Source: CAD feature listing. Evaluate the final solid. Frame: model axes, mm. Face numbers are marked on the shaded views. A direction names the side the tool comes from. Give positions to 0.01 mm unless a question says otherwise; leave off trailing zeros. Loops run counter-clockwise (first coordinate to the right, second up) from the corner with the lowest first, then second, coordinate; pieces in that order, holes last.
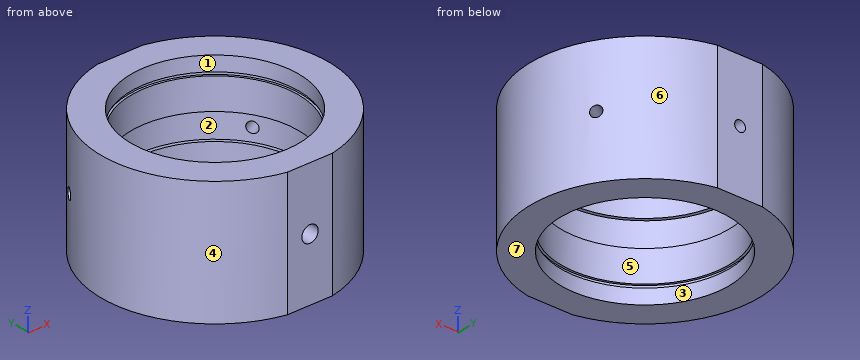
from build123d import *

# Parameters (mm, degrees)
SKETCH_2_W                       = 64.02174429
SKETCH_2_H                       = 9.248919907
CUT_EXTRUDE_1_DEPTH              = 49
HOLE_WIZARD_M4_2_D               = 3.3
HOLE_WIZARD_M4_2_DEPTH           = 5.5
HOLE_WIZARD_M4_2_TIP             = 0.991420021
HOLE_WIZARD_M6_2_D               = 5
HOLE_WIZARD_M6_2_DEPTH           = 5.5
HOLE_WIZARD_M6_2_TIP             = 1.502151548
HOLE_WIZARD_M4_3_D               = 3.3
HOLE_WIZARD_M4_3_DEPTH           = 10.1
HOLE_WIZARD_M4_3_TIP             = 0.991420021
HOLE_WIZARD_M4_3_ON_FACE_2_D     = 3.3
HOLE_WIZARD_M4_3_ON_FACE_2_DEPTH = 10.1
HOLE_WIZARD_M4_3_ON_FACE_2_TIP   = 0.991420021


with BuildPart() as part:
    # 草图1 → 旋转1 (revolve)
    with BuildSketch(Plane(origin=(0, 0, 0), x_dir=(1, 0, 0), z_dir=(0, 1, 0)), mode=Mode.PRIVATE) as revolve_1_sk:
        Polygon((34.5, 19), (34.5, -19), (25.5, -19), (25.5, -14.5), (26.1, -14.5), (26.1, -13.5), (25.4, -13.5), (25.4, -4), (26.5, -4), (26.5, 4), (25.4, 4), (25.4, 13.5), (26.1, 13.5), (26.1, 14.5), (25.5, 14.5), (25.5, 19), align=None)
    revolve(revolve_1_sk.sketch.rotate(Axis((0, 0, -31.9390681), (0, 0, 1)), 180), axis=Axis((0, 0, -31.9390681), (0, 0, 1)))  # turned: the seam where the file's is

    # 草图2 → 切除-拉伸1 (cut)
    with BuildSketch(Plane.XY.offset(19)):
        with Locations((-1.141100508, 38.424459954)):
            Rectangle(SKETCH_2_W, SKETCH_2_H)
        with Locations((-1.141100508, -38.424459954)):
            Rectangle(SKETCH_2_W, SKETCH_2_H)
    extrude(amount=-CUT_EXTRUDE_1_DEPTH, mode=Mode.SUBTRACT)

    # M4 螺纹孔2
    with Locations(Plane(origin=(0, 33.8, 0), x_dir=(1, 0, 0), z_dir=(0, 1, 0))):
        with Locations((0, 0)):
            Hole(HOLE_WIZARD_M4_2_D / 2, depth=HOLE_WIZARD_M4_2_DEPTH)
            with Locations((0, 0, -(HOLE_WIZARD_M4_2_DEPTH + HOLE_WIZARD_M4_2_TIP / 2))):  # 118° drill point
                Cone(0, HOLE_WIZARD_M4_2_D / 2, HOLE_WIZARD_M4_2_TIP, mode=Mode.SUBTRACT)

    # M6 螺纹孔2
    with Locations(Plane(origin=(0, -33.8, 0), x_dir=(-1, 0, 0), z_dir=(0, -1, 0))):
        with Locations((0, 0)):
            Hole(HOLE_WIZARD_M6_2_D / 2, depth=HOLE_WIZARD_M6_2_DEPTH)
            with Locations((0, 0, -(HOLE_WIZARD_M6_2_DEPTH + HOLE_WIZARD_M6_2_TIP / 2))):  # 118° drill point
                Cone(0, HOLE_WIZARD_M6_2_D / 2, HOLE_WIZARD_M6_2_TIP, mode=Mode.SUBTRACT)

    # M4 螺纹孔3
    with Locations(Plane(origin=(29.877876431, 17.25, 0), x_dir=(-0.5, 0.866025404, 0), z_dir=(0.866025404, 0.5, 0))):
        with Locations((0, 0)):
            Hole(HOLE_WIZARD_M4_3_D / 2, depth=HOLE_WIZARD_M4_3_DEPTH)
            with Locations((0, 0, -(HOLE_WIZARD_M4_3_DEPTH + HOLE_WIZARD_M4_3_TIP / 2))):  # 118° drill point
                Cone(0, HOLE_WIZARD_M4_3_D / 2, HOLE_WIZARD_M4_3_TIP, mode=Mode.SUBTRACT)

    # M4 螺纹孔3 on face 2
    with Locations(Plane(origin=(-29.877876431, 17.25, 0), x_dir=(-0.500000175, -0.866025303, 0), z_dir=(-0.866025303, 0.500000175, 0))):
        with Locations((0, 0)):
            Hole(HOLE_WIZARD_M4_3_ON_FACE_2_D / 2, depth=HOLE_WIZARD_M4_3_ON_FACE_2_DEPTH)
            with Locations((0, 0, -(HOLE_WIZARD_M4_3_ON_FACE_2_DEPTH + HOLE_WIZARD_M4_3_ON_FACE_2_TIP / 2))):  # 118° drill point
                Cone(0, HOLE_WIZARD_M4_3_ON_FACE_2_D / 2, HOLE_WIZARD_M4_3_ON_FACE_2_TIP, mode=Mode.SUBTRACT)


solid = part.part
1) Reachability of the marked faces 1, 2 and 3 from +Z, -Z, +X, -X, +Y, -Y: full face, straight path, thin tool, end or side. Return the list, or none.
Checks:
face 1: +Z
face 2: none
face 3: -Z
2) Pull-direction query (X, two-part tool) for the marked faces 4, 5, 6 and 7; classes: released by +X, released by -X, zero draft, split by the parting line, or undercut.
Checks:
face 4: released by -X
face 5: undercut
face 6: released by +X
face 7: zero draft
3) Ray query, probe 1 along Z at (x, y) = (0, 32.5); probe 2 along Y at (x, z) = (0, 13); probe 3 along Z at (x, y) = (-26, -4). Return the intervals inside material, ascending.
Checks:
probe 1: z = -19 to -1.65, 1.65 to 19
probe 2: y = -33.8 to -25.4, 25.4 to 33.8
probe 3: z = -19 to -4, 4 to 19
4) Contact query for flat-ended pins moving along their axis: P1, Ø6, axis at y = -7.5, z = 10.5, coming from the +X side; P2, Ø12, axis at y = -19.5, z = 8.5, coming from the -X side; P3, Ø4, axis at y = -23.5, z = -0.5, coming from the +X side. Output: stop coordinate, or through.
Checks:
P1: stops at x = 34.21
P2: stops at x = -31.75
P3: stops at x = 26.98
5) Cut plane C-C (z = -8.5). Return loops of the section in (x, y).
Checks:
outline: (-6.91, -33.8) - (6.91, -33.8) arc R34.5 ccw to (6.91, 33.8) - (-6.91, 33.8) arc R34.5 ccw to start; hole circle Ø50.8 at (0, 0)
